```python
from build123d import *

# Parameters (mm, degrees)
F2_T     = 1
F3_R     = 5.5
F4_DEPTH = 13.501


with BuildPart() as f1:
    # F0 (on Front) → F1 (revolve)
    with BuildSketch(Plane.XZ):
        with BuildLine():
            Line((0, 12.5), (0, -12.5))
            Line((0, -12.5), (67, -12.5))
            ThreePointArc((67, -12.5), (35.7561183576, 6.0463971983), (0, 12.5))
        make_face()
    revolve(axis=Axis((0, 0, 0), (0, 0, -1)))

    # F2
    f2_openings = [f1.faces().sort_by_distance(p)[0] for p in [
        (0, 0, -12.5),
    ]]
    offset(amount=F2_T, openings=f2_openings)

    # F3 (on Top) → F4 (cut, through all)
    with BuildSketch(Plane.XY):
        Circle(F3_R)
    extrude(amount=F4_DEPTH, mode=Mode.SUBTRACT)


solid = f1.part
```
The model under review builds one solid part; all positions refer to its coordinate system, in mm. Round coordinates to 2 decimals unless told otherwise and drop trailing zeros. Order: outer loops, then holes, each group sorted by start corner. A loop starts at its lowest first (then second) coordinate and runs counter-clockwise, first axis right, second up. Notation, with made-up numbers: (-13, -37) -> (43, -37) arc R24 ccw to (43, 1) -> close; hole circle Ø5 at (63.25, 2). An arc over 180 degrees is marked (long way). One line per item, written item: value. Start each with the question number.
Q1. Take a section at C-C (z = 10.25). Write out the cut boundary in (x, y).
Q2. Mouldability with a two-part tool opening along X and no side actions: class faces 1 (the face through (-1.19, -5.37, 12.85)), 2 (the face through (-66, 15, -12.5)) as released by +X, released by -X, zero draft, split by the parting line, or undercut.
Q3. Wall thickness on line 1 (Y direction, x = 0, z = -6.25); line 2 (X direction, y = 21.5, z = -1.25); line 3 (X direction, y = -50.5, z = -11.5): over which ranges is each line inside the solid? List them lowest first.
Q4. Take a section at D-D (x = 58). Write out the cut boundary in (y, z), and give its area (3 significant figures).
Q5. Clearance check with flat-ended pins moving along their axes: pin 1 Ø10 at (y, z) = (-6.5, 6.5) entering from +X; pin 2 Ø5 at (x, z) = (2.5, -9.5) entering from -Y; pin 3 Ø5 at (x, z) = (9, -4.5) entering from -Y; pin 4 Ø17.5 at (x, y) = (0, 0) entering from +Z. State where each tip first meets the part, or that it passes through.
Q6. Take a section at A-A (x = 0). Write out the cut boundary in (y, z).
Reported:
1. outline: circle Ø51.41 at (0, 0); hole circle Ø42.67 at (0, 0)
2. face 1: undercut
2. face 2: zero draft
3. line 1: y = -60.74 to -59.02, 59.02 to 60.74
3. line 2: x = -48.65 to -46.49, 46.49 to 48.65
3. line 3: x = -44.6 to -42.23, 42.23 to 44.6
4. outline: (-36.48, -12.5) -> (-33.54, -12.5) arc R84.24 cw to (33.54, -12.5) -> (36.48, -12.5) arc R85.46 ccw to start
4. area: 87.5 mm2
5. pin 1: stops at x = 47.9
5. pin 2: stops at y = -67.9
5. pin 3: stops at y = -61.12
5. pin 4: stops at z = 13.35
6. outline: (-68.52, -12.5) -> (-67, -12.5) arc R102.28 cw to (-5.5, 12.35) -> (-5.5, 13.35) arc R103.28 ccw to start; (5.5, 12.35) arc R102.28 cw to (67, -12.5) -> (68.52, -12.5) arc R103.28 ccw to (5.5, 13.35) -> close
